Read the model definition and answer for the solid it produces. Units are mm, in the model's axes. Face numbers are marked on the shaded views. A direction names the side the tool comes from. Round coordinates to 2 decimals unless told otherwise and drop trailing zeros. Write each loop counter-clockwise with the first axis right and the second up, starting at its lowest first coordinate (ties: lowest second). Pieces come first, ordered by that corner, then holes. Notation, with made-up numbers: (-9, -4.5) -> (29, -4.5) arc R19 cw to (29, 21.5) -> close; hole circle Ø11 at (-15, 37.5). An arc over 180 degrees is marked (long way). Return JSON: item names as keys, results as strings.
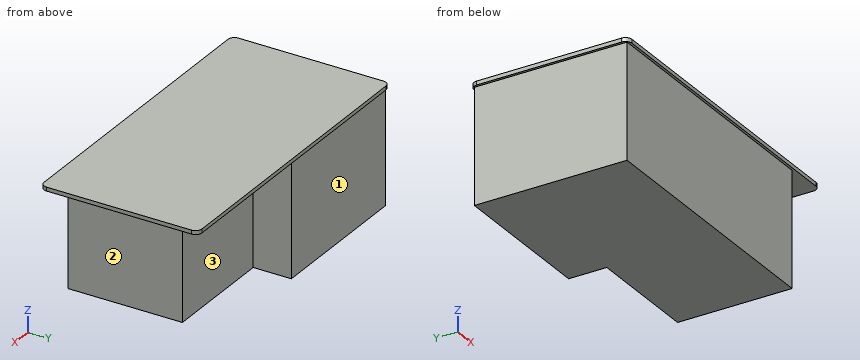
from build123d import *

# Parameters (mm, degrees)
F0_W     = 2400
F0_H     = 1200
F1_DEPTH = 900
F2_W     = 2440
F2_H     = 1240
F3_DEPTH = 30
F4_W     = 300
F4_H     = 300
F4_W_2   = 900
F4_H_2   = 900
F5_DEPTH = 900
F6_R     = 50


with BuildPart() as f1:
    # F0 (on Top) → F1 (new body)
    with BuildSketch(Plane.XY):
        with Locations((11.786235, -165.532895)):
            Rectangle(F0_W, F0_H)
    extrude(amount=F1_DEPTH)

    # F2 (on face) → F3 (join)
    with BuildSketch(Plane.XY.offset(900)):
        with Locations((11.786235, -165.532895)):
            Rectangle(F2_W, F2_H)
    extrude(amount=F3_DEPTH)

    # F4 (on face) → F5 (cut)
    with BuildSketch(Plane(origin=(0, 0, 0), x_dir=(1, 0, 0), z_dir=(0, 0, -1))):
        with Locations((1061.786235, -284.467105)):
            Rectangle(F4_W, F4_H)
        with Locations((461.786235, -284.467105)):
            Rectangle(F4_W_2, F4_H)
        with Locations((1061.786235, 315.532895)):
            Rectangle(F4_W, F4_H_2)
    extrude(amount=-F5_DEPTH, mode=Mode.SUBTRACT)

    # F6
    f6_edges = [f1.edges().sort_by_distance(p)[0] for p in [
        (1231.786235, 454.467105, 915),
        (1231.786235, -785.532895, 915),
        (-1208.213765, 454.467105, 915),
        (-1208.213765, -785.532895, 915),
    ]]
    fillet(f6_edges, radius=F6_R)


solid = f1.part
Item 1: Section B-B (y = 368.5) is taken. Give the vertices of the cut face in (x, z).
Worked answers:
{"outline": "(-1208.21, 900) -> (-1188.21, 900) -> (-1188.21, 0) -> (11.79, 0) -> (11.79, 900) -> (1231.79, 900) -> (1231.79, 930) -> (-1208.21, 930) -> close"}
Item 2: Section A-A (x = -206) is taken. Give the vertices of the cut face in (y, z), then the cut area to 3 significant figures.
Worked answers:
{"outline": "(-785.53, 900) -> (-765.53, 900) -> (-765.53, 0) -> (434.47, 0) -> (434.47, 900) -> (454.47, 900) -> (454.47, 930) -> (-785.53, 930) -> close", "area": "1,120,000 mm2"}
Item 3: Straight lines are drawn through the part: L1, parallel to Y at x = -285, z = 395; L2, parallel to X at y = -556, z = 469.5; L3, parallel to Y at x = 703.5, z = 710.5. For each, find the intervals that lie inside material, in ascending order. Write a range as [from, to].
Worked answers:
{"L1": "y = [-765.53, 434.47]", "L2": "x = [-1188.21, 911.79]", "L3": "y = [-765.53, 134.47]"}
Item 4: A tool of negligible diameter and unlimited length cuts with its end or side. For the marked faces 1, 2 and 3, from which of +Z, -Z, +X, -X, +Y, -Y can it reach the whole face along a straight path? Write none if from no direction.
Worked answers:
{"face 1": "-Z, +X, -X, +Y", "face 2": "-Z, +X, +Y, -Y", "face 3": "-Z, +X, +Y"}
Item 5: Section C-C (z = 444) is taken. Give the vertices of the cut face in (x, y), then the cut area to 3 significant figures.
Worked answers:
{"outline": "(-1188.21, -765.53) -> (911.79, -765.53) -> (911.79, 134.47) -> (11.79, 134.47) -> (11.79, 434.47) -> (-1188.21, 434.47) -> close", "area": "2,250,000 mm2"}
Item 6: Flat-ended cylindrical pins translate along their axes: pin 1 (1 mm diameter, centred on x = -564.5, z = 428.5, fed in from +Y); pin 2 (5 mm diameter, centred on x = 721.5, z = 392, fed in from -Y); pin 3 (1 mm diameter, centred on y = 309.5, z = 300.5, fed in from -X). Find the tip coordinate at first contact, or state that the pin passes through.
Worked answers:
{"pin 1": "stops at y = 434.47", "pin 2": "stops at y = -765.53", "pin 3": "stops at x = -1188.21"}
